```python
from build123d import *

# Parameters (mm, degrees)
F0_W     = 230
F0_H     = 114
F1_DEPTH = 76
F3_W     = 20
F3_H     = 76
F4_DEPTH = 230.001
F6_W     = 38
F6_H     = 20
F7_DEPTH = 114.001


with BuildPart() as f1:
    # F0 (on Front) → F1 (new body)
    with BuildSketch(Plane.XZ):
        Rectangle(F0_W, F0_H)
    extrude(amount=F1_DEPTH)

    # F3 (on offset) → F4 (cut, through all)
    with BuildSketch(Plane.YZ.offset(115)):
        with Locations((-10, 19)):
            Rectangle(F3_W, F3_H)
    extrude(amount=-F4_DEPTH, mode=Mode.SUBTRACT)

    # F6 (on offset) → F7 (cut, through all)
    with BuildSketch(Plane.XY.offset(-57)):
        with Locations((-96, -10)):
            Rectangle(F6_W, F6_H)
        with Locations((96, -10)):
            Rectangle(F6_W, F6_H)
    extrude(amount=F7_DEPTH, mode=Mode.SUBTRACT)


solid = f1.part
```
Could you check a few things on this model? Use its own coordinates, in mm. A direction names the side the tool comes from. Coordinates: 2 decimals unless noted, no trailing zeros. Order: outer loops, then holes, each group sorted by start corner. A loop starts at its lowest first (then second) coordinate and runs counter-clockwise, first axis right, second up. Notation, with made-up numbers: M -34.75,-40 L -5.75,-40 A35 ccw -5.75,-7 Z; hole C 82.25,35.5 d11. An arc over 180 degrees is marked long. Use one line per item in the form item = value. Start each with the question number.
1. On a 3-axis mill with a long thin cutter (end or side, diameter ignored), from which of +Z, -Z, +X, -X, +Y, -Y can I reach the whole of each face in a straight line? I mean faces 1 (the flat face through (-77, -10, -38)), 2 (the flat face through (-115, -48, -1)), 3 (the flat face through (77, -10, -38)), 4 (the flat face through (1, -10, -19)), 5 (the flat face through (-2, -37, -57)). Say none if no direction works.
2. Suppose I cut it at D-D on x = -91.5. Write out the boundary of the cut face in (y, z), then the cut area to 3 significant figures.
3. Suppose I cut it at C-C on y = -11. Write out the boundary of the cut face in (x, z), then the cut area to 3 significant figures.
4. For pin 1 (6 mm diameter, centred on y = -12.5, z = -29.5, fed in from -X); pin 2 (16 mm diameter, centred on x = 9, y = -14, fed in from +Z); pin 3 (6 mm diameter, centred on y = -11, z = -43.5, fed in from +X), each with a flat end and sliding along its axis, tell me the tip position at first contact or that it passes through.
5. Please list where these lines run through material, in increasing order: line 1 (Z direction, x = 33, y = -16.5); line 2 (Y direction, x = 103.5, z = 23.5).
6. Suppose I cut it at B-B on x = 63. Write out the boundary of the cut face in (y, z).
7. Suppose I cut it at A-A on z = -29. Write out the boundary of the cut face in (x, y).
Geometry says:
q1.face_1 = +Z, -Z, -X, +Y
q1.face_2 = +Z, -Z, -X, +Y, -Y
q1.face_3 = +Z, -Z, +X, +Y
q1.face_4 = +Z, +X, -X, +Y
q1.face_5 = -Z, +X, -X, +Y, -Y
q2.outline = M -76,-57 L -20,-57 L -20,57 L -76,57 Z
q2.area = 6,380 mm^2
q3.outline = M -77,-57 L 77,-57 L 77,-19 L -77,-19 Z
q3.area = 5,850 mm^2
q4.pin_1 = -77
q4.pin_2 = 57
q4.pin_3 = 77
q5.line_1 = -57 to -19
q5.line_2 = -76 to -20
q6.outline = M -76,-57 L 0,-57 L 0,-19 L -20,-19 L -20,57 L -76,57 Z
q7.outline = M -115,-76 L 115,-76 L 115,-20 L 77,-20 L 77,0 L -77,0 L -77,-20 L -115,-20 Z
